Geometry: final body of the model. Coordinates: model frame, mm. Give positions to 0.01 mm unless a question says otherwise; leave off trailing zeros. Answer in a Markdown table with one row per item. Add a question column.
Item 1: Section query A-A on z = 1.75. State how many separate pieces and enclosed holes the cut face has, plus the area to 3 significant figures.
Item 2: First-contact query: P1, Ø0.9, axis at y = 2.5, z = 1, coming from the -X side; P2, Ø0.9, axis at x = 101.5, z = 1.5, coming from the -Y side. Flat tips, straight axial feed; report the tip coordinate or a pass-through.
Item 3: Material intervals for probe 1 along X at (y, z) = (5.5, 0.2); probe 2 along X at (y, z) = (41, 0.9); probe 3 along Y at (x, z) = (272.5, 1.25), sorted ascending. Write a range as from..to.
```python
from build123d import *

# Parameters (mm, degrees)
ESQUISSE1_R        = 1.5
BOSS_EXTRU_1_DEPTH = 3
CONG_1_R           = 4


with BuildPart() as part:
    # Esquisse1 → Boss.-Extru.1 (new body)
    with BuildSketch(Plane.XY):
        Polygon((0, 0), (0, 45), (5, 45), (5, 37.5), (10, 37.5), (10, 45), (100, 45), (100, 37.5), (105, 37.5), (105, 45), (130, 45), (130, 25), (150, 25), (150, 45), (175, 45), (175, 37.5), (180, 37.5), (180, 45), (270, 45), (270, 37.5), (275, 37.5), (275, 45), (280, 45), (280, 0), (275, 0), (275, 7.5), (270, 7.5), (270, 0), (180, 0), (180, 7.5), (175, 7.5), (175, 0), (105, 0), (105, 7.5), (100, 7.5), (100, 0), (10, 0), (10, 7.5), (5, 7.5), (5, 0), align=None)
        with Locations((7.5, 22.5)):
            Circle(ESQUISSE1_R, mode=Mode.SUBTRACT)
        with Locations((102.5, 22.5)):
            Circle(ESQUISSE1_R, mode=Mode.SUBTRACT)
        with Locations((177.5, 22.5)):
            Circle(ESQUISSE1_R, mode=Mode.SUBTRACT)
        with Locations((272.5, 22.5)):
            Circle(ESQUISSE1_R, mode=Mode.SUBTRACT)
    extrude(amount=BOSS_EXTRU_1_DEPTH)

    # Congé1
    cong_1_edges = [part.edges().sort_by_distance(p)[0] for p in [
        (0, 0, 1.5),
        (0, 45, 1.5),
        (130, 45, 1.5),
        (130, 25, 1.5),
        (150, 25, 1.5),
        (150, 45, 1.5),
        (280, 45, 1.5),
        (280, 0, 1.5),
    ]]
    fillet(cong_1_edges, radius=CONG_1_R)


solid = part.part
```
Findings below:
| question | item | result |
|---|---|---|
| 1 | separate pieces | 1 |
| 1 | enclosed holes | 4 |
| 1 | area | 11,900 mm^2 |
| 2 | P1 | stops at x = 0.14 |
| 2 | P2 | stops at y = 7.5 |
| 3 | probe 1 | x = 0..5, 10..100, 105..175, 180..270, 275..280 |
| 3 | probe 2 | x = 0..5, 10..100, 105..130, 150..175, 180..270, 275..280 |
| 3 | probe 3 | y = 7.5..21, 24..37.5 |
